For this review, take the finished solid that the model builds, in its own axes (mm). A direction names the side the tool comes from. Round coordinates to 2 decimals unless told otherwise and drop trailing zeros. Write each loop counter-clockwise with the first axis right and the second up, starting at its lowest first coordinate (ties: lowest second). Pieces come first, ordered by that corner, then holes.
from build123d import *

# Parameters (mm, degrees)
PAD_DEPTH       = 0.4
SKETCH001_R     = 2
POCKET_DEPTH    = 5
PAD001_DEPTH    = 6
POCKET001_DEPTH = 6.401
FILLET_R        = 0.5
FILLET001_R     = 0.39
FILLET002_R     = 0.9


with BuildPart() as part:
    # Sketch → Pad (new body)
    with BuildSketch(Plane.XY):
        with BuildLine():
            Line((-32.7, 6.275), (32.7, 6.275))
            ThreePointArc((34.7, 4.275), (34.114214, 5.689214), (32.7, 6.275))
            Line((34.7, 4.275), (34.7, -4.275))
            ThreePointArc((32.7, -6.275), (34.114214, -5.689214), (34.7, -4.275))
            Line((32.7, -6.275), (-32.7, -6.275))
            ThreePointArc((-34.7, -4.275), (-34.114214, -5.689214), (-32.7, -6.275))
            Line((-34.7, -4.275), (-34.7, 4.275))
            ThreePointArc((-32.7, 6.275), (-34.114214, 5.689214), (-34.7, 4.275))
        make_face()
    extrude(amount=PAD_DEPTH)

    # Sketch001 (on Face10 of Pad) → Pocket (cut)
    with BuildSketch(Plane.XY.offset(0.4)):
        with Locations((-31.755, 0)):
            Circle(SKETCH001_R)
        with Locations((31.755, 0)):
            Circle(SKETCH001_R)
    extrude(amount=-POCKET_DEPTH, mode=Mode.SUBTRACT)

    # Sketch002 (on Face5 of Pocket) → Pad001 (join)
    with BuildSketch(Plane.XY.offset(0.4)):
        with BuildLine():
            Line((-25.11, 4.6), (25.11, 4.6))
            ThreePointArc((28.064304, 1.078381), (27.408354, 3.5281), (25.11, 4.6))
            Line((28.064304, 1.078381), (27.499304, -2.121619))
            ThreePointArc((24.545, -4.6), (26.4731, -3.898354), (27.499304, -2.121619))
            Line((24.545, -4.6), (-24.545, -4.6))
            ThreePointArc((-27.499304, -2.121619), (-26.4731, -3.898354), (-24.545, -4.6))
            Line((-27.499304, -2.121619), (-28.064304, 1.078381))
            ThreePointArc((-25.11, 4.6), (-27.408354, 3.5281), (-28.064304, 1.078381))
        make_face()
    extrude(amount=PAD001_DEPTH)

    # Sketch003 (on Face21 of Pad001) → Pocket001 (cut, through all)
    with BuildSketch(Plane.XY.offset(6.4)):
        with BuildLine():
            Line((-25.11, 4.2), (25.11, 4.2))
            ThreePointArc((27.670397, 1.14793), (27.101906, 3.27102), (25.11, 4.2))
            Line((27.670397, 1.14793), (27.105397, -2.05207))
            ThreePointArc((24.545, -4.2), (26.21602, -3.591906), (27.105397, -2.05207))
            Line((24.545, -4.2), (-24.545, -4.2))
            ThreePointArc((-27.105397, -2.05207), (-26.21602, -3.591906), (-24.545, -4.2))
            Line((-27.105397, -2.05207), (-27.670397, 1.14793))
            ThreePointArc((-25.11, 4.2), (-27.101906, 3.27102), (-27.670397, 1.14793))
        make_face()
    extrude(amount=-POCKET001_DEPTH, mode=Mode.SUBTRACT)

    # Fillet
    fillet_edges = [part.edges().sort_by_distance(p)[0] for p in [
        (0, -4.6, 0.4),
    ]]
    fillet(fillet_edges, radius=FILLET_R)

    # Fillet001
    fillet001_edges = [part.edges().sort_by_distance(p)[0] for p in [
        (-26.4731, -3.898354, 6.4),
    ]]
    fillet(fillet001_edges, radius=FILLET001_R)

    # Fillet002
    fillet002_edges = [part.edges().sort_by_distance(p)[0] for p in [
        (0, 4.2, 0),
    ]]
    fillet(fillet002_edges, radius=FILLET002_R)


solid = part.part
(1) We need section A-A, the plane x = 19. Give the boundary of the cut face in (y, z) (3 decimals).
Geometry check:
outline: (-6.275, 0) - (-5.1, 0) arc R0.9 ccw to (-4.2, 0.9) - (-4.2, 6.4) - (-4.21, 6.4) arc R0.39 ccw to (-4.6, 6.01) - (-4.6, 0.9) arc R0.5 cw to (-5.1, 0.4) - (-6.275, 0.4) - close; (4.2, 0.9) arc R0.9 ccw to (5.1, 0) - (6.275, 0) - (6.275, 0.4) - (5.1, 0.4) arc R0.5 cw to (4.6, 0.9) - (4.6, 6.01) arc R0.39 ccw to (4.21, 6.4) - (4.2, 6.4) - close
(2) For line 1 along Y through (x, z) = (17, 1.75); line 2 along X through (y, z) = (3.5, 3.5); line 3 along X through (y, z) = (0.25, 2.5), list the stretches that pass through material, from the lowest coordinate up.
Geometry check:
line 1: y = -4.6 to -4.2, 4.2 to 4.6
line 2: x = -27.43 to -26.88, 26.88 to 27.43
line 3: x = -27.92 to -27.51, 27.51 to 27.92
(3) We need section B-B, the plane y = 0. State how many separate pieces and enclosed holes the cut face has, and give its area (3 significant figures).
Geometry check:
separate pieces: 4
enclosed holes: 0
area: 7.15 mm2
(4) Mouldability with a two-part tool opening along X and no side actions: class faces 1 (the face through (-26.495, -3.879, 3.419)), 2 (the face through (34.099, -5.705, 0.197)), 3 (the face through (-33.753, 0.088, 0.203)) as pulls with the +X half, pulls with the -X half, needs draft (parallel to the pull), parting line crosses it, or undercut.
Geometry check:
face 1: pulls with the -X half
face 2: pulls with the +X half
face 3: undercut
(5) For faces 4 (the face through (0, 4.6, 3)), 5 (the face through (26.45, -3.92, 3.42)), 6 (the face through (-27.384, -0.474, 3.688)), 7 (the face through (-27.64, -0.52, 0.27)), list the 3-axis set-ups (+Z, -Z, +X, -X, +Y, -Y) from which the entire face can be reached by the end or side of a thin tool; tool diameter is ignored.
Geometry check:
face 4: +Z, +X, -X, +Y
face 5: +Z, +X, -Y
face 6: +Z, -Z
face 7: -Z
(6) For pin 1 Ø4 at (x, y) = (-22.5, 2) entering from -Z; pin 2 Ø1.5 at (x, z) = (-27, 2.5) entering from -Y; pin 3 Ø3 at (x, z) = (-1.5, 3) entering from +Y; pin 4 Ø1 at (y, z) = (4, 1.5) entering from -X, all flat-tipped, find the tip position at first contact; note any pin that passes through.
Geometry check:
pin 1: passes through
pin 2: stops at y = -4.07
pin 3: stops at y = 4.6
pin 4: stops at x = -27.43
